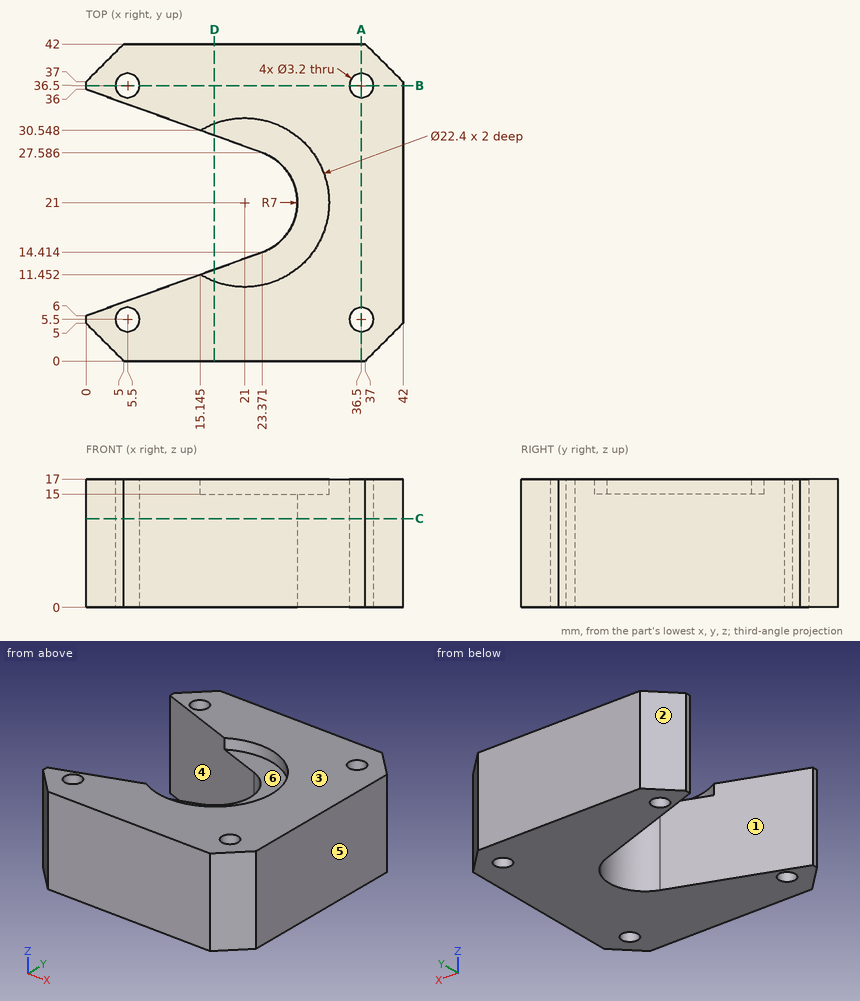
Geometry: see drawing. Coordinates: mm, zero at the bounding-box minimum. A direction names the side the tool comes from. Round coordinates to 2 decimals unless told otherwise and drop trailing zeros. Order: outer loops, then holes, each group sorted by start corner. A loop starts at its lowest first (then second) coordinate and runs counter-clockwise, first axis right, second up. Notation, with made-up numbers: (-23.5, 44) - (11.5, 44) arc R16 ccw to (11.5, 60) - close; hole circle Ø7 at (-4.75, 32.5). An arc over 180 degrees is marked (long way). One line per question, with ' | ' between items. Start each with the question number.
1) Cut plane C-C, the plane z = 11.75. Return the cut outline in (x, y), then the cut area to 3 significant figures.
2) Pull-direction query (X, two-part tool) for the marked faces 3, 4, 5 and 6; classes: +X half, -X half, draft (parallel to the pull), parting line (faces both ways), or undercut.
3) Cut plane D-D, the plane x = 17. Return the cut outline in (y, z).
4) Ray query, probe 1 along Y at (x, z) = (36.5, 3.5); probe 2 along Y at (x, z) = (5.5, 5.5); probe 3 along Y at (x, z) = (6, 5). Return the intervals inside material, ascending.
5) Cut plane A-A, the plane x = 36.5. Return the cut outline in (y, z), then the cut area to 3 significant figures.
6) Set-up query: the marked faces 1 and 2. Return all of +Z, -Z, +X, -X, +Y, -Y with unobstructed straight access to the full face (end or side cutting, diameter ignored); none if empty.
7) Contact query for a flat-ended pin moving along its axis: P1, Ø6, axis at x = 27.5, y = 24.5, coming from the +Z side. Output: stop coordinate, or through.
Worked out:
1) outline: (0, 5) - (5, 0) - (37, 0) - (42, 5) - (42, 37) - (37, 42) - (5, 42) - (0, 37) - (0, 36) - (23.37, 27.59) arc R7 cw to (23.37, 14.41) - (0, 6) - close; hole circle Ø3.2 at (5.5, 5.5); hole circle Ø3.2 at (5.5, 36.5); hole circle Ø3.2 at (36.5, 5.5); hole circle Ø3.2 at (36.5, 36.5) | area: 1,130 mm^2
2) face 3: draft | face 4: -X half | face 5: +X half | face 6: undercut
3) outline: (0, 0) - (12.12, 0) - (12.12, 15) - (10.54, 15) - (10.54, 17) - (0, 17) - close; (29.88, 0) - (42, 0) - (42, 17) - (31.46, 17) - (31.46, 15) - (29.88, 15) - close
4) probe 1: y = 0 to 3.9, 7.1 to 34.9, 38.1 to 42 | probe 2: y = 0 to 3.9, 7.1 to 7.98, 34.02 to 34.9, 38.1 to 42 | probe 3: y = 0 to 3.98, 7.02 to 8.16, 33.84 to 34.98, 38.02 to 42
5) outline: (0, 0) - (3.9, 0) - (3.9, 17) - (0, 17) - close; (7.1, 0) - (34.9, 0) - (34.9, 17) - (7.1, 17) - close; (38.1, 0) - (42, 0) - (42, 17) - (38.1, 17) - close | area: 605 mm^2
6) face 1: +Z, -Z, -X | face 2: +Z, -Z, -X, +Y
7) P1: stops at z = 15
